Model file for the job. Use its own axes, mm. A direction names the side the tool comes from. Round coordinates to 2 decimals unless told otherwise and drop trailing zeros. Order: outer loops, then holes, each group sorted by start corner. A loop starts at its lowest first (then second) coordinate and runs counter-clockwise, first axis right, second up. Notation, with made-up numbers: (70, -20) - (113, -20) arc R29 cw to (113, 14) - close; hole circle Ø9 at (-6.75, -34.75). An arc over 180 degrees is marked (long way). Write item = value, one per line.
```python
from build123d import *

# Parameters (mm, degrees)
SKETCH1_R           = 0.889
BOSS_EXTRUDE1_DEPTH = 12.7
SKETCH2_R           = 0.508
CUT_EXTRUDE1_DEPTH  = 12.7


with BuildPart() as part:
    # Sketch1 → Boss-Extrude1 (new body)
    with BuildSketch(Plane.XY):
        with BuildLine():
            Line((-20.6375, -7.688584311), (-20.6375, 7.567266813))
            Line((-20.6375, 7.567266813), (20.6375, 7.567266813))
            Line((20.6375, 7.567266813), (20.6375, -7.688584311))
            ThreePointArc((20.6375, -7.688584311), (16.525068691, -20.050967212), (5.826741818, -27.486450005))
            ThreePointArc((5.826741818, -27.486450005), (4.931277216, -27.325327691), (4.523886836, -26.511785848))
            Line((4.523886836, -26.511785848), (4.523886836, -24.938668143))
            ThreePointArc((4.523886836, -24.938668143), (4.821466346, -24.220247653), (5.539886836, -23.922668143))
            Line((5.539886836, -23.922668143), (6.102813797, -23.922668143))
            ThreePointArc((6.102813797, -23.922668143), (6.78239506, -23.641176367), (7.063886836, -22.961595104))
            Line((7.063886836, -22.961595104), (7.063886836, -21.519985546))
            Line((7.063886836, -21.519985546), (8.481348217, -20.102524164))
            ThreePointArc((8.481348217, -20.102524164), (8.689682664, -19.79072963), (8.762839993, -19.422942901))
            Line((8.762839993, -19.422942901), (8.762839993, -17.898886311))
            ThreePointArc((8.762839993, -17.898886311), (11.420440685, -14.802736841), (13.027769559, -11.052339947))
            ThreePointArc((13.027769559, -11.052339947), (13.455022544, -7.688584311), (13.027769559, -4.324828675))
            ThreePointArc((13.027769559, -4.324828675), (0, 5.766438233), (-13.027769559, -4.324828675))
            ThreePointArc((-13.027769559, -4.324828675), (-13.455022544, -7.688584311), (-13.027769559, -11.052339947))
            ThreePointArc((-13.027769559, -11.052339947), (-11.420440685, -14.802736841), (-8.762839993, -17.898886311))
            Line((-8.762839993, -17.898886311), (-8.762839993, -19.422942901))
            ThreePointArc((-8.762839993, -19.422942901), (-8.689682664, -19.79072963), (-8.481348217, -20.102524164))
            Line((-8.481348217, -20.102524164), (-7.063886836, -21.519985546))
            Line((-7.063886836, -21.519985546), (-7.063886836, -22.961595104))
            ThreePointArc((-7.063886836, -22.961595104), (-6.78239506, -23.641176367), (-6.102813797, -23.922668143))
            Line((-6.102813797, -23.922668143), (-5.539886836, -23.922668143))
            ThreePointArc((-5.539886836, -23.922668143), (-4.821466346, -24.220247653), (-4.523886836, -24.938668143))
            Line((-4.523886836, -24.938668143), (-4.523886836, -26.511785848))
            ThreePointArc((-4.523886836, -26.511785848), (-4.931277216, -27.325327691), (-5.826741818, -27.486450005))
            ThreePointArc((-5.826741818, -27.486450005), (-16.525068691, -20.050967212), (-20.6375, -7.688584311))
        make_face()
        with Locations((-17.5, -7.688584311)):
            Circle(SKETCH1_R, mode=Mode.SUBTRACT)
        with Locations((17.5, -7.688584311)):
            Circle(SKETCH1_R, mode=Mode.SUBTRACT)
    extrude(amount=BOSS_EXTRUDE1_DEPTH)

    # Sketch2 → Cut-Extrude1 (cut)
    with BuildSketch(Plane(origin=(0, 7.567266813, 0), x_dir=(1, 0, 0), z_dir=(0, 1, 0))):
        with Locations(Location((-17.5, -6.35, 0), (0, 0, 270))):
            Circle(SKETCH2_R)
        with Locations(Location((17.5, -6.35, 0), (0, 0, 270))):
            Circle(SKETCH2_R)
    extrude(amount=-CUT_EXTRUDE1_DEPTH, mode=Mode.SUBTRACT)


solid = part.part
```
1) Cut at A-A (z = 1.5). Write the cut outline in (x, y) (1 decimal), and give its area (3 significant figures).
Conclusion:
outline = (-20.6, -7.7) arc R20.6 ccw to (-5.8, -27.5) arc R1 ccw to (-4.5, -26.5) - (-4.5, -24.9) arc R1 ccw to (-5.5, -23.9) - (-6.1, -23.9) arc R1 cw to (-7.1, -23) - (-7.1, -21.5) - (-8.5, -20.1) arc R1 cw to (-8.8, -19.4) - (-8.8, -17.9) arc R13.5 cw (long way) to (8.8, -17.9) - (8.8, -19.4) arc R1 cw to (8.5, -20.1) - (7.1, -21.5) - (7.1, -23) arc R1 cw to (6.1, -23.9) - (5.5, -23.9) arc R1 ccw to (4.5, -24.9) - (4.5, -26.5) arc R1 ccw to (5.8, -27.5) arc R20.6 ccw to (20.6, -7.7) - (20.6, 7.6) - (-20.6, 7.6) - close; hole circle Ø1.8 at (-17.5, -7.7); hole circle Ø1.8 at (17.5, -7.7)
area = 630 mm^2
2) Wall check: line 1 along X through (y, z) = (-2.25, 6.35); line 2 along X through (y, z) = (-8, 10.25); line 3 along X through (y, z) = (2.5, 4). Give the ranges that are in metal, low to high.
Conclusion:
line_1 = -20.64 to -18.01, -16.99 to -12.31, 12.31 to 16.99, 18.01 to 20.64
line_2 = -20.64 to -18.33, -16.67 to -13.45, 13.45 to 16.67, 18.33 to 20.64
line_3 = -20.64 to -8.79, 8.79 to 20.64
3) Cut at B-B (y = 2). Write the cut outline in (x, z).
Conclusion:
outline = (-20.64, 0) - (-9.34, 0) - (-9.34, 12.7) - (-20.64, 12.7) - close; (9.34, 0) - (20.64, 0) - (20.64, 12.7) - (9.34, 12.7) - close; hole circle Ø1.02 at (-17.5, 6.35); hole circle Ø1.02 at (17.5, 6.35)
4) Cut at D-D (x = 17.5). Write the cut outline in (y, z), and give its area (3 significant figures).
Conclusion:
outline = (-18.63, 0) - (-8.58, 0) - (-8.58, 12.7) - (-18.63, 12.7) - close; (-6.8, 0) - (7.57, 0) - (7.57, 5.84) - (-5.13, 5.84) - (-5.13, 6.86) - (7.57, 6.86) - (7.57, 12.7) - (-6.8, 12.7) - close
area = 297 mm^2
5) Cut at C-C (y = -12). Write the cut outline in (x, z).
Conclusion:
outline = (-20.18, 0) - (-12.75, 0) - (-12.75, 12.7) - (-20.18, 12.7) - close; (12.75, 0) - (20.18, 0) - (20.18, 12.7) - (12.75, 12.7) - close
6) 3-axis set-ups, long thin cutter, end or side, ignore diameter. For faces 5 (the face through (-17.5, -5.133, 6.3)), 6 (the face through (-4.524, -26, 6)), 7 (the face through (7.064, -22, 6)), 8 (the face through (-20.638, 0, 6)): which of +Z, -Z, +X, -X, +Y, -Y reach the whole face in a straight line?
Conclusion:
face_5 = +Y
face_6 = +Z, -Z, -Y
face_7 = +Z, -Z
face_8 = +Z, -Z, -X, +Y, -Y
7) Flat gauge pins, fed straight in: pin 1 Ø5 at (x, y) = (-5.5, -0.5) entering from -Z; pin 2 Ø1.1 at (x, z) = (-17.5, 6.5) entering from +Y; pin 3 Ø0.5 at (y, z) = (-26, 8.5) entering from +X; pin 4 Ø0.7 at (y, z) = (-22, 3.5) entering from -X. Where does each tip first touch, or does it go through?
Conclusion:
pin_1 = through
pin_2 = 7.57
pin_3 = 9.98
pin_4 = -15.2
8) Mould opens along Y. For faces 1 (the face through (4.81, -24.23, 6.26)), 2 (the face through (17.5, -5.133, 6.3)), 3 (the face through (-16.413, -20.199, 6.261)), 4 (the face through (4.524, -26, 6)) say: +Y half, -Y half, draft (parallel to the pull), parting line (faces both ways), or undercut.
Conclusion:
face_1 = undercut
face_2 = +Y half
face_3 = -Y half
face_4 = draft
